```python
from build123d import *

# Parameters (mm, degrees)
F1_DEPTH = 6


with BuildPart() as f1:
    # F0 (on Top) → F1 (new body)
    with BuildSketch(Plane.XY):
        with BuildLine():
            Line((250, 0), (0, 0))
            Line((0, 0), (0, -155))
            Line((0, -155), (110.4873499226, -86.497843048))
            add(Edge.make_bspline(
                [(110.4873499226, -86.497843048), (107.2843735439, -77.0023074484), (131.9373436968, -61.4037722235), (163.3322021719, -41.7004632777), (169.9805383425, -49.6120662277)],
                knots=[0, 0, 0, 0, 0.2195299732, 0.4558974308, 0.4558974308, 0.4558974308, 0.4558974308], degree=3))
            Line((169.9805383425, -49.6120662277), (250, 0))
        make_face()
        with BuildLine():
            Line((20, -89.3357885437), (20, -40))
            ThreePointArc((20, -40), (25.8578643763, -25.8578643763), (40, -20))
            Line((40, -20), (125.702884748, -20))
            ThreePointArc((125.702884748, -20), (135.3203238346, -27.2604990574), (130.9722814366, -38.4990269171))
            Line((130.9722814366, -38.4990269171), (35.2693966886, -97.8348154609))
            ThreePointArc((35.2693966886, -97.8348154609), (25.1365632977, -98.0734646331), (20, -89.3357885437))
        make_face(mode=Mode.SUBTRACT)
    extrude(amount=-F1_DEPTH)


solid = f1.part
```
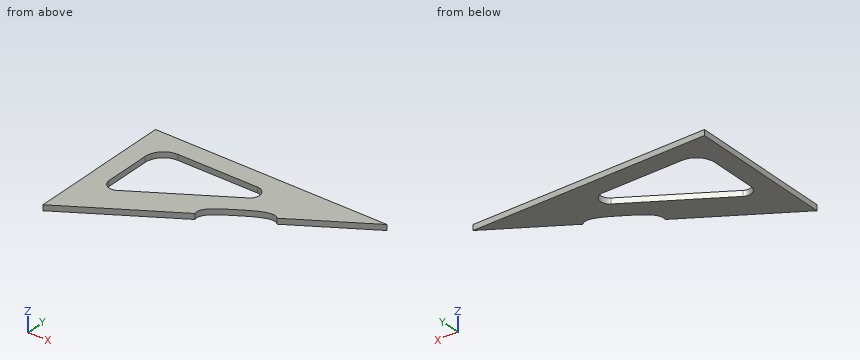
Model file for the job. Use its own axes, mm. Coordinates: 2 decimals unless noted, no trailing zeros. Loops run counter-clockwise (first coordinate to the right, second up) from the corner with the lowest first, then second, coordinate; pieces in that order, holes last. Notation, with made-up numbers: (-23, 32) -> (0, 32) arc R10 cw to (0, 46) -> close; hole circle Ø6 at (-5.75, 64). An arc over 180 degrees is marked (long way). Answer as a JSON object with one key per item and string values.
Q1. Cut at A-A (x = 16.5). List the corners of the cut face in (y, z), and give its area (3 significant figures).
Report:
{"outline": "(-144.77, -6) -> (0, -6) -> (0, 0) -> (-144.77, 0) -> close", "area": "869 mm2"}
Q2. Probe probe 1 along X at (y, z) = (-59, -1.5); probe 2 along Y at (x, z) = (75.5, -4); probe 3 along X at (y, z) = (-90, -2.5). List the from-to ranges inside material, lowest first.
Report:
{"probe 1": "x = 0 to 20, 97.91 to 135.82", "probe 2": "y = -108.19 to -72.89, -20 to 0", "probe 3": "x = 0 to 20.02, 47.91 to 104.84"}
Q3. Cut at B-B (y = -15.5). List the corners of the cut face in (x, z), and give its area (3 significant figures).
Report:
{"outline": "(0, -6) -> (225, -6) -> (225, 0) -> (0, 0) -> close", "area": "1,350 mm2"}
Q4. Flat gauge pins, fed straight in: P1, Ø2, axis at x = 84, z = -4.5, coming from the -Y side; P2, Ø3, axis at y = -45, z = -1.5, coming from the +X side; P3, Ø3, axis at x = 79.5, z = -2.5, coming from the -Y side. Where does each tip first touch, or does it go through?
Report:
{"P1": "stops at y = -103.54", "P2": "stops at x = 179.84", "P3": "stops at y = -106.64"}
